The drawing under review shows one solid part. Ordinate dimensions are in mm from its lowest x, y, z. Round coordinates to 2 decimals unless told otherwise and drop trailing zeros. Order: outer loops, then holes, each group sorted by start corner. A loop starts at its lowest first (then second) coordinate and runs counter-clockwise, first axis right, second up. Notation, with made-up numbers: M 47,28.25 L 81,28.25 A25 cw 81,49.25 Z; hole C -7,48 d2. An arc over 180 degrees is marked long. Answer as a JSON object with one key per item and string values. Group by question number.
1) To check wall thickness, follow line 1 (Y direction, x = 4.75, z = 12); line 2 (Z direction, x = 4.75, y = 4.25); line 3 (Y direction, x = 2.5, z = 12). State the ranges of each line that lie inside material, in increasing order.
2) Insertion check: pin 1 Ø3 at (x, z) = (7, 120.5) entering from -Y; pin 2 Ø2 at (y, z) = (2.5, 69) entering from +X. Each pin has a flat end and moves straight along its axis. Give the tip position at first contact, or say it passes through.
3) Consider section A-A, the plane y = 4.5. Write out the cut boundary in (x, z), then the cut area to 3 significant figures.
4) Consider section D-D, the plane z = 56. Write out the cut boundary in (x, y), then the cut area to 3 significant figures.
5) Consider section B-B, the plane x = 2.5. Write out the cut boundary in (y, z).
6) Consider section C-C, the plane z = 12. Write out the cut boundary in (x, y), then the cut area to 3 significant figures.
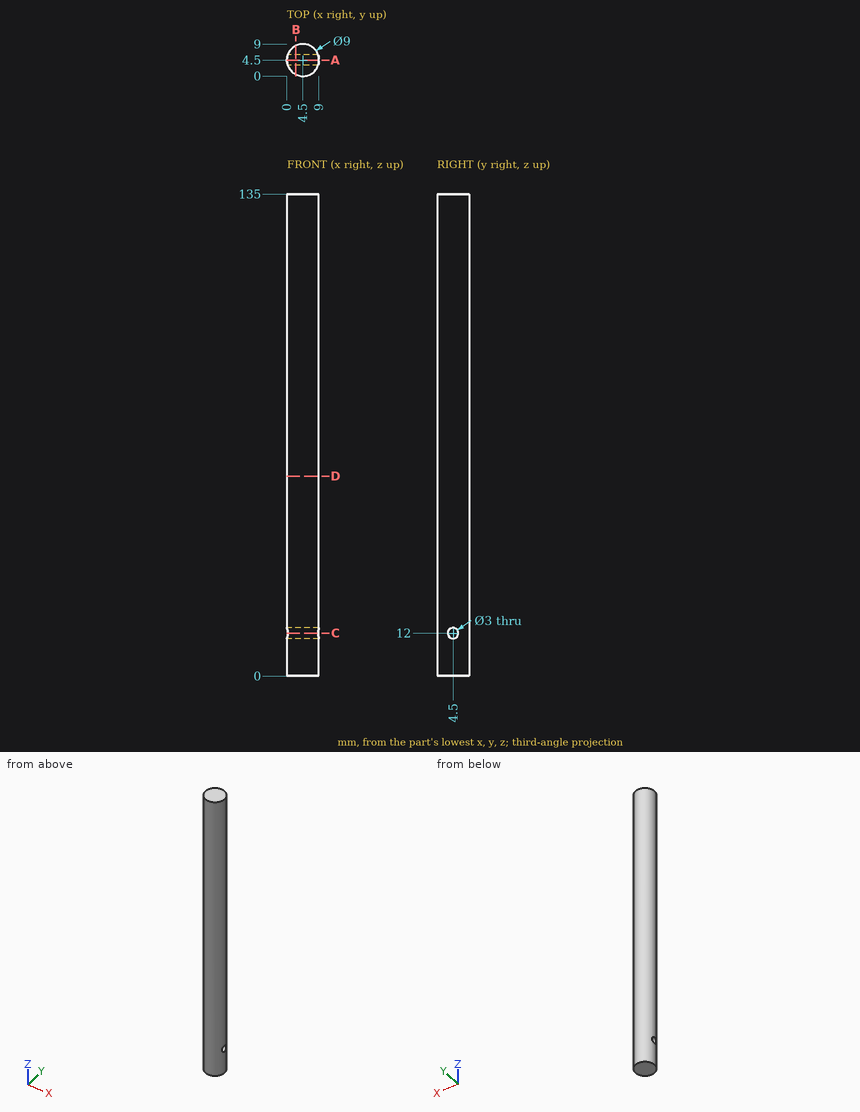
Results list:
{
 "1": {"line 1": "0.01 to 3, 6 to 8.99", "line 2": "0 to 10.52, 13.48 to 135", "line 3": "0.47 to 3, 6 to 8.53"},
 "2": {"pin 1": "y = 0.11", "pin 2": "x = 8.89"},
 "3": {"outline": "M 0,0 L 9,0 L 9,10.5 L 0,10.5 Z; M 0,13.5 L 9,13.5 L 9,135 L 0,135 Z", "area": "1,190 mm^2"},
 "4": {"outline": "C 4.5,4.5 d9", "area": "63.6 mm^2"},
 "5": {"outline": "M 0.47,0 L 8.53,0 L 8.53,135 L 0.47,135 Z; hole C 4.5,12 d3"},
 "6": {"outline": "M 0.26,3 A4.5 ccw 8.74,3 Z; M 0.26,6 L 8.74,6 A4.5 ccw Z", "area": "37.1 mm^2"}
}
